Drawing for the job (mm, zero at the part's lowest x, y, z). A direction names the side the tool comes from. Round coordinates to 2 decimals unless told otherwise and drop trailing zeros. Write each loop counter-clockwise with the first axis right and the second up, starting at its lowest first coordinate (ties: lowest second). Pieces come first, ordered by that corner, then holes. Notation, with made-up numbers: (45, -7) - (91, -7) arc R16 cw to (91, 18) - close; hole circle Ø11 at (15.5, -18.75). An arc over 180 degrees is marked (long way). Answer in a Markdown table with one row per item.
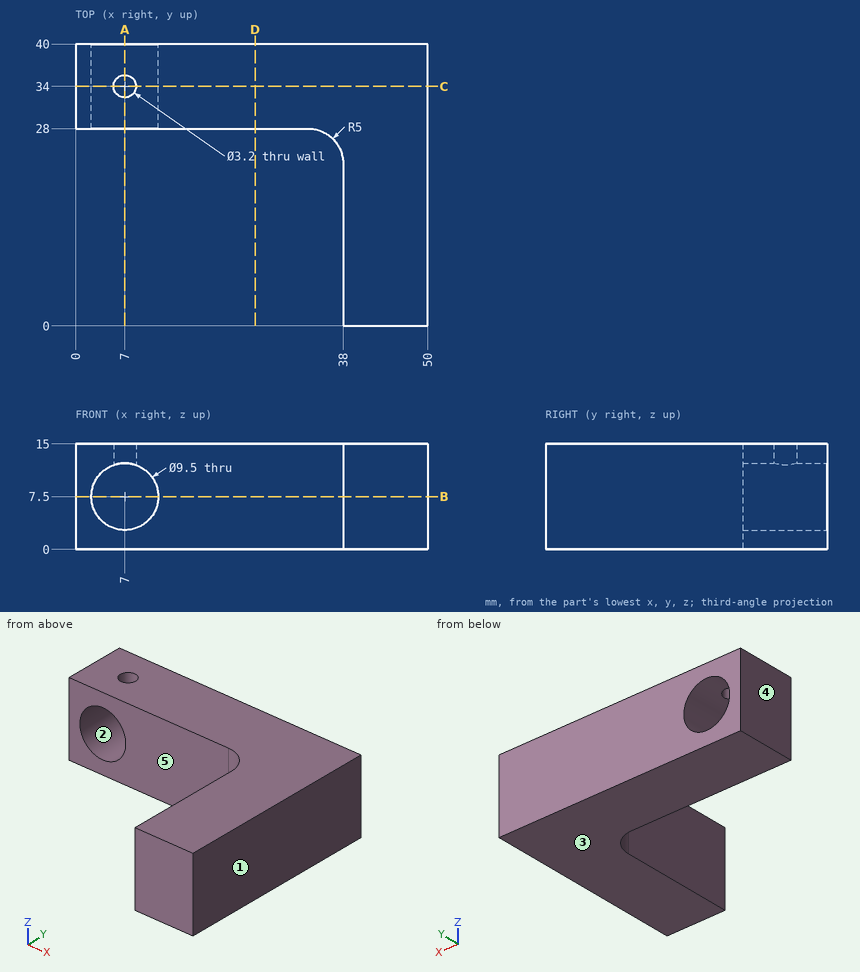
Q1. Drill centre lines: line 1 (X direction, y = 34, z = 13.5); line 2 (Z direction, x = 7, y = 31); line 3 (Y direction, x = 7, z = 13.95). Where is each one in solid material? Low to high.
Computed:
| item | result |
|---|---|
| line 1 | x = 0 to 5.4, 8.6 to 50 |
| line 2 | z = 0 to 2.75, 12.25 to 15 |
| line 3 | y = 28 to 32.4, 35.6 to 40 |
Q2. Saw through at A-A on x = 7. List the corners of the cut face in (y, z), then the cut area to 3 significant figures.
Computed:
| item | result |
|---|---|
| outline | (28, 0) - (40, 0) - (40, 2.75) - (28, 2.75) - close; (28, 12.25) - (32.4, 12.25) - (32.4, 15) - (28, 15) - close; (35.6, 12.25) - (40, 12.25) - (40, 15) - (35.6, 15) - close |
| area | 57.2 mm2 |
Q3. Saw through at B-B on z = 7.5. List the corners of the cut face in (x, y), then the cut area to 3 significant figures.
Computed:
| item | result |
|---|---|
| outline | (0, 28) - (2.25, 28) - (2.25, 40) - (0, 40) - close; (11.75, 28) - (33, 28) arc R5 cw to (38, 23) - (38, 0) - (50, 0) - (50, 40) - (11.75, 40) - close |
| area | 827 mm2 |
Q4. Saw through at C-C on y = 34. List the corners of the cut face in (x, z), then the cut area to 3 significant figures.
Computed:
| item | result |
|---|---|
| outline | (0, 0) - (50, 0) - (50, 15) - (8.6, 15) - (8.6, 11.97) arc R4.75 cw (long way) to (5.4, 11.97) - (5.4, 15) - (0, 15) - close |
| area | 670 mm2 |
Q5. 3-axis set-ups, long thin cutter, end or side, ignore diameter. For the marked faces 4 and 5: which of +Z, -Z, +X, -X, +Y, -Y reach the whole face in a straight line?
Computed:
| item | result |
|---|---|
| face 4 | +Z, -Z, -X, +Y, -Y |
| face 5 | +Z, -Z, -X, -Y |
Q6. Pull direction Z, two halves, no side cores. Call the marked faces 1, 2 and 3: released by +Z, released by -Z, zero draft, split by the parting line, or undercut.
Computed:
| item | result |
|---|---|
| face 1 | zero draft |
| face 2 | undercut |
| face 3 | released by -Z |
Q7. Saw through at D-D on x = 25.5. List the corners of the cut face in (y, z), then the cut area to 3 significant figures.
Computed:
| item | result |
|---|---|
| outline | (28, 0) - (40, 0) - (40, 15) - (28, 15) - close |
| area | 180 mm2 |
Q8. Flat gauge pins, fed straight in: pin 1 (1 mm diameter, centred on x = 9.5, z = 4, fed in from +Y); pin 2 (10 mm diameter, centred on x = 25, y = 19, fed in from +Z); pin 3 (1 mm diameter, centred on x = 12.5, z = 3, fed in from -Y). Where does each tip first touch, or does it go through?
Computed:
| item | result |
|---|---|
| pin 1 | stops at y = 40 |
| pin 2 | passes through |
| pin 3 | stops at y = 28 |
